Could you check a few things on this drawing? It's one solid part, dimensions in mm from its lowest x, y, z. A direction names the side the tool comes from. Give positions to 0.01 mm unless a question says otherwise; leave off trailing zeros. Order: outer loops, then holes, each group sorted by start corner. A loop starts at its lowest first (then second) coordinate and runs counter-clockwise, first axis right, second up. Notation, with made-up numbers: (37.5, 77.5) - (91.5, 77.5) arc R9 ccw to (91.5, 94.5) - close; hole circle Ø9 at (79.25, -37.75). An arc over 180 degrees is marked (long way). Put each result on its own line as item: value.
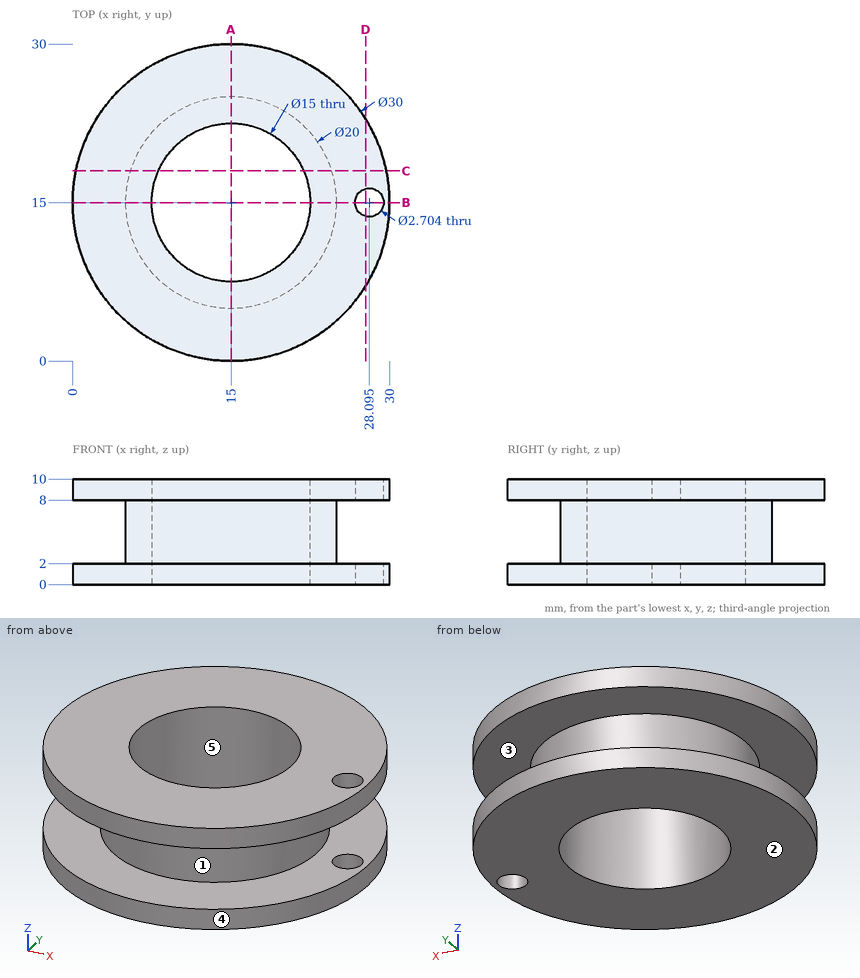
1) Which directions (+Z, -Z, +X, -X, +Y, -Y) give clear straight access to the entire face, cutting with the end or side of a thin tool? Please do the marked faces 1 and 2.
Filled in:
face 1: none
face 2: -Z, +X, -X, +Y, -Y
2) If I drill on line 1 (Z direction, x = 9.5, y = 4); line 2 (X direction, y = 14.75, z = 8.25) (1 decimal); line 3 (Y direction, x = 12.25, z = 9.25) (1 decimal), over which ranges is the centre line in solid material (lowest first)? Write a range as [from, to].
Filled in:
line 1: z = [0, 2], [8, 10]
line 2: x = [0, 7.5], [22.5, 26.8], [29.4, 30]
line 3: y = [0.3, 8], [22, 29.7]
3) Suppose I cut it at A-A, the plane x = 15. List the corners of the cut face in (y, z) for me.
Filled in:
outline: (0, 0) - (7.5, 0) - (7.5, 10) - (0, 10) - (0, 8) - (5, 8) - (5, 2) - (0, 2) - close; (22.5, 0) - (30, 0) - (30, 2) - (25, 2) - (25, 8) - (30, 8) - (30, 10) - (22.5, 10) - close
4) I'm going to push flat-ended pins straight in: pin 1 (1 mm diameter, centred on x = 24, y = 7.5, fed in from -Z); pin 2 (3 mm diameter, centred on y = 26.5, z = 8, fed in from -X); pin 3 (2 mm diameter, centred on x = 17, z = 5.5, fed in from -Y). Where does each tip first touch, or does it pass through?
Filled in:
pin 1: stops at z = 0
pin 2: stops at x = 3.82
pin 3: stops at y = 5.05
5) Suppose I cut it at D-D, the plane x = 27.75. List the corners of the cut face in (y, z) for me.
Filled in:
outline: (7.1, 0) - (13.69, 0) - (13.69, 2) - (7.1, 2) - close; (7.1, 8) - (13.69, 8) - (13.69, 10) - (7.1, 10) - close; (16.31, 0) - (22.9, 0) - (22.9, 2) - (16.31, 2) - close; (16.31, 8) - (22.9, 8) - (22.9, 10) - (16.31, 10) - close
6) Suppose I cut it at B-B, the plane y = 15. List the corners of the cut face in (x, z) for me.
Filled in:
outline: (0, 0) - (7.5, 0) - (7.5, 10) - (0, 10) - (0, 8) - (5, 8) - (5, 2) - (0, 2) - close; (22.5, 0) - (26.74, 0) - (26.74, 2) - (25, 2) - (25, 8) - (26.74, 8) - (26.74, 10) - (22.5, 10) - close; (29.45, 0) - (30, 0) - (30, 2) - (29.45, 2) - close; (29.45, 8) - (30, 8) - (30, 10) - (29.45, 10) - close
7) Suppose I cut it at C-C, the plane y = 18. List the corners of the cut face in (x, z) for me.
Filled in:
outline: (0.3, 0) - (8.13, 0) - (8.13, 10) - (0.3, 10) - (0.3, 8) - (5.46, 8) - (5.46, 2) - (0.3, 2) - close; (21.87, 0) - (29.7, 0) - (29.7, 2) - (24.54, 2) - (24.54, 8) - (29.7, 8) - (29.7, 10) - (21.87, 10) - close
8) We'd pull the mould along X, two halves only. Please class the marked faces 3, 4 and 5: pulls with the +X half, pulls with the -X half, needs draft (parallel to the pull), parting line crosses it, or undercut.
Filled in:
face 3: needs draft
face 4: parting line crosses it
face 5: undercut
